Source: three-view drawing plus pictorial views. Frame: mm from the lowest corner of the part. A direction names the side the tool comes from. Give positions to 0.01 mm unless a question says otherwise; leave off trailing zeros. Loops run counter-clockwise (first coordinate to the right, second up) from the corner with the lowest first, then second, coordinate; pieces in that order, holes last. Notation, with made-up numbers: (25.25, 68.5) -> (81.25, 68.5) arc R32 ccw to (81.25, 96.5) -> close; hole circle Ø8 at (17.25, 17). An arc over 180 degrees is marked (long way). Answer in a Markdown table with one row per item. Add a question column.
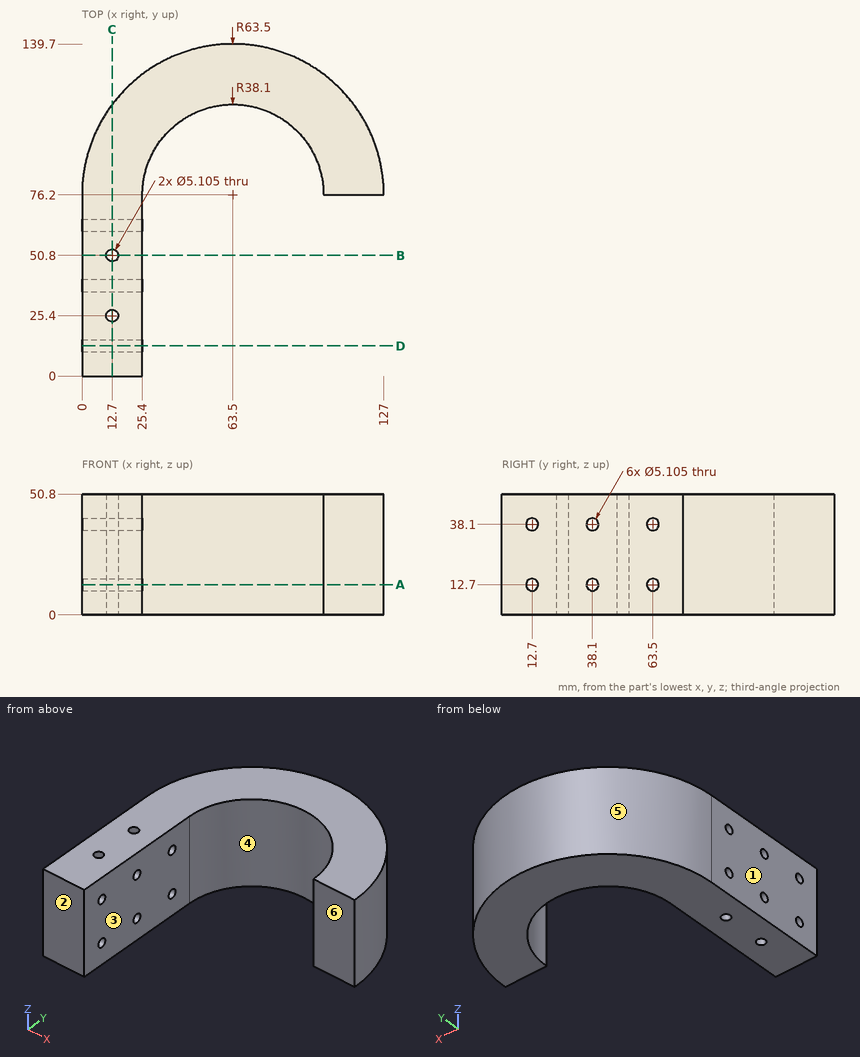
(1) Cut plane A-A on z = 12.7. Return the cut outline in (x, y) (1 decimal).
(2) Cut plane D-D on y = 12.7. Return the cut outline in (x, z).
(3) Cut plane B-B on y = 50.8. Return the cut outline in (x, z).
(4) Reachability of the marked faces 5 and 6 from +Z, -Z, +X, -X, +Y, -Y: full face, straight path, thin tool, end or side. Return the list, or none.
(5) Draft query along X for the marked faces 1, 2, 3 and 4. Return one class per face: +X half, -X half, draft (parallel to the pull), parting line (faces both ways), or undercut.
(6) Pin query (flat end, axial travel): pin 1 Ø4 at (y, z) = (63.5, 12.7) entering from -X; pin 2 Ø8 at (y, z) = (38.1, 38.1) entering from +X; pin 3 Ø3 at (x, z) = (24, 21.5) entering from +Y (1 decimal); pin 4 Ø1.5 at (x, z) = (34, 38.5) entering from +Y. Return the tip coordinate at first contact, or that it passes through.
(7) Material intervals for line 1 along Y through (x, z) = (15.75, 12.7) (1 decimal); line 2 along Y through (x, z) = (18, 38.1) (1 decimal); line 3 along X through (y, z) = (111.5, 15.5) (1 decimal), sorted ascending. Write a range as from..to.
(8) Cut plane C-C on x = 12.7. State how many separate pieces and enclosed holes the cut face has.
Answer list:
| question | item | result |
|---|---|---|
| 1 | outline | (0, 0) -> (25.4, 0) -> (25.4, 10.1) -> (0, 10.1) -> close; (0, 15.3) -> (25.4, 15.3) -> (25.4, 35.5) -> (0, 35.5) -> close; (0, 40.7) -> (25.4, 40.7) -> (25.4, 60.9) -> (0, 60.9) -> close; (0, 66.1) -> (25.4, 66.1) -> (25.4, 76.2) arc R38.1 cw to (101.6, 76.2) -> (127, 76.2) arc R63.5 ccw to (0, 76.2) -> close; hole circle Ø5.1 at (12.7, 25.4); hole circle Ø5.1 at (12.7, 50.8) |
| 2 | outline | (0, 0) -> (25.4, 0) -> (25.4, 10.15) -> (0, 10.15) -> close; (0, 15.25) -> (25.4, 15.25) -> (25.4, 35.55) -> (0, 35.55) -> close; (0, 40.65) -> (25.4, 40.65) -> (25.4, 50.8) -> (0, 50.8) -> close |
| 3 | outline | (0, 0) -> (10.15, 0) -> (10.15, 50.8) -> (0, 50.8) -> close; (15.25, 0) -> (25.4, 0) -> (25.4, 50.8) -> (15.25, 50.8) -> close |
| 4 | face 5 | +Z, -Z, +Y |
| 4 | face 6 | +Z, -Z, +X, -Y |
| 5 | face 1 | -X half |
| 5 | face 2 | draft |
| 5 | face 3 | +X half |
| 5 | face 4 | undercut |
| 6 | pin 1 | passes through |
| 6 | pin 2 | stops at x = 25.4 |
| 6 | pin 3 | stops at y = 127.1 |
| 6 | pin 4 | stops at y = 132.82 |
| 7 | line 1 | y = 0..10.1, 15.3..35.5, 40.7..60.9, 66.1..118.1 |
| 7 | line 2 | y = 0..10.1, 15.3..35.5, 40.7..60.9, 66.1..120.5 |
| 7 | line 3 | x = 10.7..49.2, 77.8..116.3 |
| 8 | separate pieces | 3 |
| 8 | enclosed holes | 6 |
